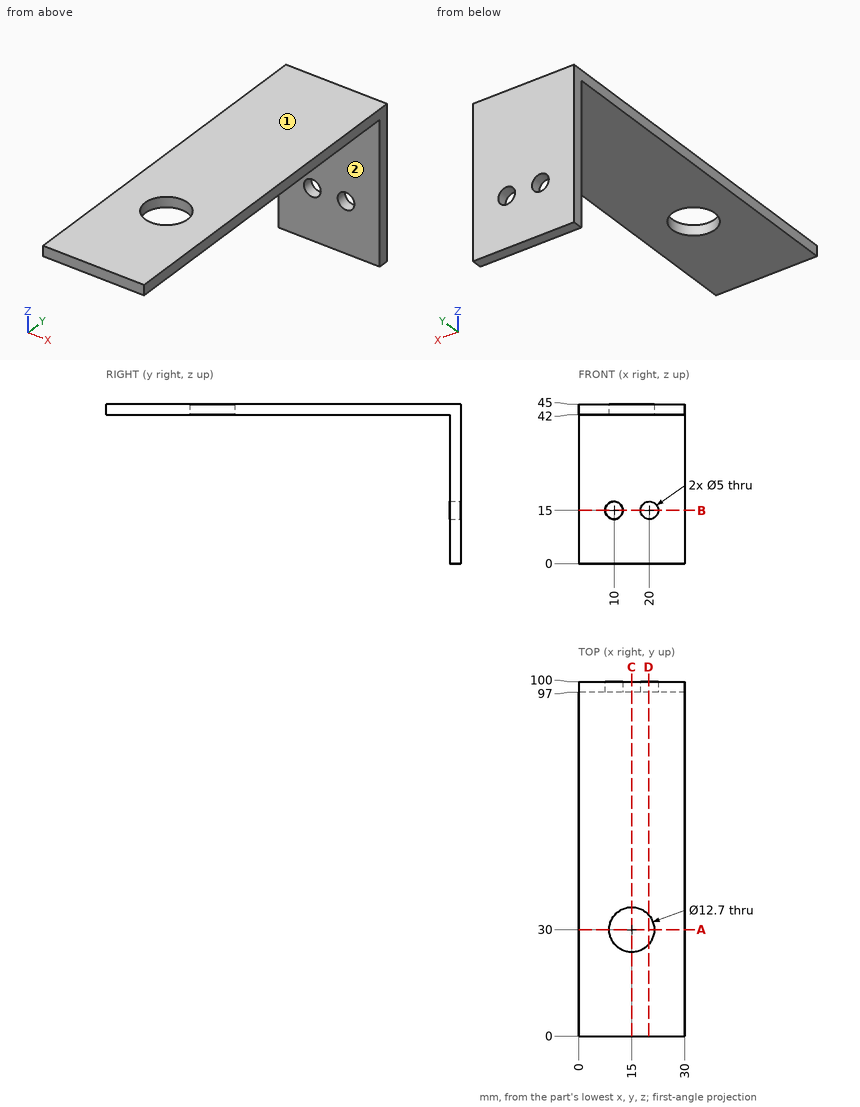
Input: dimensioned drawing with shaded views. Units: mm. Origin: part minimum x, y, z. A direction names the side the tool comes from. Give positions to 0.01 mm unless a question says otherwise; leave off trailing zeros. Write each loop counter-clockwise with the first axis right and the second up, starting at its lowest first coordinate (ties: lowest second). Pieces come first, ordered by that corner, then holes.
1. Section query D-D, the plane x = 19.75. Return loops of the section in (y, z).
2. Reachability of the marked faces 1 and 2 from +Z, -Z, +X, -X, +Y, -Y: full face, straight path, thin tool, end or side. Return the list, or none.
3. Pin query (flat end, axial travel): P1, Ø2, axis at x = 15.5, z = 33, coming from the -Y side; P2, Ø16.5, axis at x = 15, y = 30, coming from the -Z side. Return the tip coordinate at first contact, or that it passes through.
4. Line query: probe 1 along X at (y, z) = (99, 15); probe 2 along Z at (x, y) = (10, 99.35); probe 3 along Y at (x, z) = (18, 3). Output: solid intervals per line, ascending.
5. Section query C-C, the plane x = 15. Return loops of the section in (y, z).
6. Section query A-A, the plane y = 30. Return loops of the section in (x, z), then the cut area to 3 significant figures.
7. Section query B-B, the plane z = 15. Return loops of the section in (x, y), then the cut area to 3 significant figures.
Computed:
1. outline: (0, 42) - (25.79, 42) - (25.79, 45) - (0, 45) - close; (34.21, 42) - (97, 42) - (97, 17.49) - (100, 17.49) - (100, 45) - (34.21, 45) - close; (97, 0) - (100, 0) - (100, 12.51) - (97, 12.51) - close
2. face 1: +Z, +X, -X, +Y, -Y
2. face 2: -Z, +X, -X, -Y
3. P1: stops at y = 97
3. P2: stops at z = 42
4. probe 1: x = 0 to 7.5, 12.5 to 17.5, 22.5 to 30
4. probe 2: z = 0 to 12.5, 17.5 to 45
4. probe 3: y = 97 to 100
5. outline: (0, 42) - (23.65, 42) - (23.65, 45) - (0, 45) - close; (36.35, 42) - (97, 42) - (97, 0) - (100, 0) - (100, 45) - (36.35, 45) - close
6. outline: (0, 42) - (8.65, 42) - (8.65, 45) - (0, 45) - close; (21.35, 42) - (30, 42) - (30, 45) - (21.35, 45) - close
6. area: 51.9 mm2
7. outline: (0, 97) - (7.5, 97) - (7.5, 100) - (0, 100) - close; (12.5, 97) - (17.5, 97) - (17.5, 100) - (12.5, 100) - close; (22.5, 97) - (30, 97) - (30, 100) - (22.5, 100) - close
7. area: 60.0 mm2
